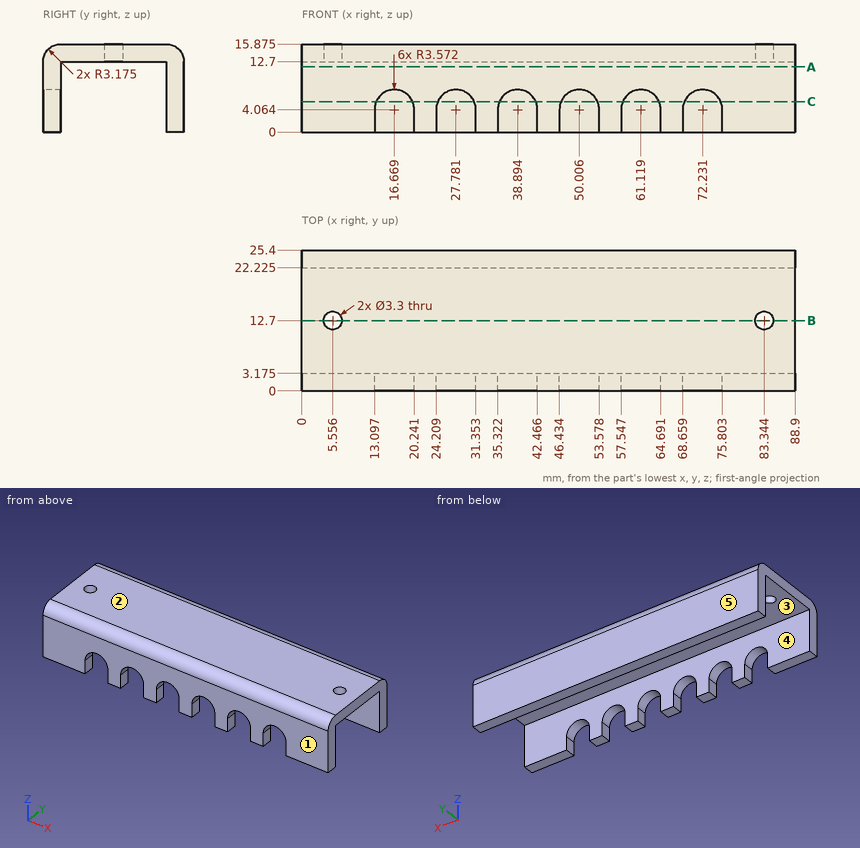
Check sheet for the drawn part. Datum: minimum x, y, z corner. Units: mm. A direction names the side the tool comes from. Coordinates: 2 decimals unless noted, no trailing zeros. Write each loop counter-clockwise with the first axis right and the second up, starting at its lowest first coordinate (ties: lowest second). Pieces come first, ordered by that corner, then holes. Notation, with made-up numbers: (-3.75, 8) - (19.25, 8) arc R6 ccw to (19.25, 13) - close; hole circle Ø4 at (24.5, -15). An arc over 180 degrees is marked (long way). Answer as a JSON object with one key per item and string values.
(1) Mould release check, pull along Y, two halves, no side actions. Record for the marked faces 1, 2 and 3: pulls with the +Y half, pulls with the -Y half, needs draft (parallel to the pull), parting line crosses it, or undercut.
Report:
{"face 1": "pulls with the -Y half", "face 2": "needs draft", "face 3": "undercut"}
(2) Cross-section at A-A on z = 11.75. Record the cut outline in (x, y) (1 decimal).
Report:
{"outline": "(0, 0) - (88.9, 0) - (88.9, 3.2) - (0, 3.2) - close; (0, 22.2) - (88.9, 22.2) - (88.9, 25.4) - (0, 25.4) - close"}
(3) Gauge pin test, flat ends, axial feed: pin 1 Ø5.5 at (x, y) = (43.5, 8) entering from -Z; pin 2 Ø1 at (x, z) = (63.5, 2) entering from -Y (3 decimals). Record the tip position at first contact, or that the pin passes through.
Report:
{"pin 1": "z = 12.7", "pin 2": "y = 22.225"}
(4) Tool access check on the marked faces 4 and 5. Record the directions out of +Z, -Z, +X, -X, +Y, -Y that give a thin tool (end or side, any length) a straight path to the whole face; none if there is none.
Report:
{"face 4": "-Z, +X, -X", "face 5": "+Z, -Z, +X, -X, +Y"}
(5) Thickness scan on line 1 along Y through (x, z) = (9, 11) (1 decimal); line 2 along Z through (x, y) = (16, 10.5) (1 decimal); line 3 along Y through (x, z) = (18.5, 4.75) (1 decimal). Record the ranges inside material, lowest first.
Report:
{"line 1": "0 to 3.2, 22.2 to 25.4", "line 2": "12.7 to 15.9", "line 3": "22.2 to 25.4"}
(6) Cross-section at C-C on z = 5.5. Give the number of separate pieces and of enclosed holes in the cut face, plus the area to 3 significant figures.
Report:
{"separate pieces": "8", "enclosed holes": "0", "area": "440 mm^2"}
(7) Cross-section at B-B on y = 12.7. Record the cut outline in (x, z) (1 decimal), plus the area to 3 significant figures.
Report:
{"outline": "(0, 12.7) - (3.9, 12.7) - (3.9, 15.9) - (0, 15.9) - close; (7.2, 12.7) - (81.7, 12.7) - (81.7, 15.9) - (7.2, 15.9) - close; (85, 12.7) - (88.9, 12.7) - (88.9, 15.9) - (85, 15.9) - close", "area": "261 mm^2"}
